Can you work these out from the model? Positions are in its coordinate system, mm. A direction names the side the tool comes from. Give positions to 0.01 mm unless a question says otherwise; leave off trailing zeros. Write each loop counter-clockwise with the first axis right and the second up, starting at its lowest first coordinate (ties: lowest second). Pieces come first, ordered by that corner, then holes. Notation, with made-up numbers: (60.25, 64) - (93.25, 64) arc R17 ccw to (93.25, 80) - close; hole circle Ø7 at (50, 2). An arc over 180 degrees is marked (long way). Use a Markdown table: item, result. Add a question column.
```python
from build123d import *

# Parameters (mm, degrees)
SKETCH1_R           = 18
BOSS_EXTRUDE1_DEPTH = 32.6
SKETCH2_R           = 1.6
CUT_EXTRUDE1_DEPTH  = 42.361334601
CIRPATTERN1_COUNT   = 8
SKETCH3_R           = 11
BOSS_EXTRUDE2_DEPTH = 2
SKETCH4_R           = 4
BOSS_EXTRUDE3_DEPTH = 16
CUT_EXTRUDE2_START  = -15
CUT_EXTRUDE2_DEPTH  = 15


with BuildPart() as part:
    # Sketch1 → Boss-Extrude1 (new body)
    with BuildSketch(Plane.XY):
        Circle(SKETCH1_R)
    extrude(amount=BOSS_EXTRUDE1_DEPTH)

    # Sketch2 → Cut-Extrude1 (cut, through all)
    with BuildSketch(Plane(origin=(0, 0, 0), x_dir=(-1, 0, 0), z_dir=(0, 0, -1))):
        with Locations((0, 14)):
            Circle(SKETCH2_R)
    cut_extrude1 = extrude(amount=-CUT_EXTRUDE1_DEPTH, mode=Mode.SUBTRACT)

    # CirPattern1: Cut-Extrude1 ×8 about axis
    cirpattern1_axis = Axis((0, 0, 0), (0, 0, 1))
    for i in range(1, CIRPATTERN1_COUNT):
        add(cut_extrude1.rotate(cirpattern1_axis, i * 360 / CIRPATTERN1_COUNT), mode=Mode.SUBTRACT)

    # Sketch3 → Boss-Extrude2 (add)
    with BuildSketch(Plane(origin=(0, 0, 0), x_dir=(-1, 0, 0), z_dir=(0, 0, -1))):
        with Locations(Location((0, 0, 0), (0, 0, 180))):
            Circle(SKETCH3_R)
    extrude(amount=BOSS_EXTRUDE2_DEPTH)

    # Sketch4 → Boss-Extrude3 (add)
    with BuildSketch(Plane(origin=(0, 0, -2), x_dir=(-1, 0, 0), z_dir=(0, 0, -1))):
        Circle(SKETCH4_R)
    extrude(amount=BOSS_EXTRUDE3_DEPTH)

    # Sketch5 → Cut-Extrude2 (cut)
    with BuildSketch(Plane(origin=(0, 0, -18), x_dir=(-1, 0, 0), z_dir=(0, 0, -1)).offset(CUT_EXTRUDE2_START)):
        with BuildLine():
            Line((-2.645751311, 3), (2.645751311, 3))
            ThreePointArc((2.645751311, 3), (0, 4), (-2.645751311, 3))
        make_face()
        with BuildLine():
            Line((-2.645751311, -3), (2.645751311, -3))
            ThreePointArc((2.645751311, -3), (0, -4), (-2.645751311, -3))
        make_face()
    extrude(amount=CUT_EXTRUDE2_DEPTH, mode=Mode.SUBTRACT)


solid = part.part
```
Q1. If we mould it in two halves opening along X, with no side actions, what happens to faces 6 (the cylindrical face through (-8.374, -9.418, 16.072)), 7 (the flat face through (0, 0, 32.6)), 8 (the cylindrical face through (-9.418, 8.374, 16.072)), 9 (the cylindrical face through (-2.343, 17.847, 16.072))? For each: released by +X, released by -X, zero draft, split by the parting line, or undercut.
Q2. I'm going to push flat-ended pins straight in: P1, Ø4, axis at x = 9.9, y = 9.9, coming from the -Z side; P2, Ø1.5, axis at y = 13, z = 0, coming from the +X side; P3, Ø0.8, axis at x = 0, y = -3.5, coming from the -Z side. Where does each tip first touch, or does it pass through?
Q3. Suppose I cut it at B-B (x = 0). Please give me the cut outline in (y, z), and give its area (3 significant figures).
Q4. If I drill on probe 1 along Y at (x, z) = (0, 10); probe 2 along Y at (x, z) = (0.5, 22); probe 3 along Z at (x, y) = (-5.5, 3), over which ranges is the centre line in solid material (lowest first)? Write a range as [from, to].
Q5. Suppose I cut it at A-A (y = 0). Please give me the cut outline in (x, z), and give its area (3 significant figures).
Q6. On a 3-axis mill with a long thin cutter (end or side, diameter ignored), from which of +Z, -Z, +X, -X, +Y, -Y can I reach the whole of each face in a straight line? I mean faces 1 (the cylindrical face through (-0.208, -15.586, 16.072)), 2 (the flat face through (0, -3, -10)), 3 (the flat face through (0, 0, -18)), 4 (the flat face through (0, 3, -10)), 5 (the flat face through (0, 5, -2)). Say none if no direction works.
Q7. Suppose I cut it at C-C (z = 14). Give the number of separate pieces and of enclosed holes in the cut face, and give its area (3 significant figures).
Q8. Suppose I cut it at D-D (x = -14). Please give me the cut outline in (y, z), and give its area (3 significant figures).
Derived:
| question | item | result |
|---|---|---|
| 1 | face 6 | undercut |
| 1 | face 7 | zero draft |
| 1 | face 8 | undercut |
| 1 | face 9 | split by the parting line |
| 2 | P1 | z = 0 |
| 2 | P2 | x = 13.19 |
| 2 | P3 | z = -3 |
| 3 | outline | (-18, 0) - (-15.6, 0) - (-15.6, 32.6) - (-18, 32.6) - close; (-12.4, 0) - (-11, 0) - (-11, -2) - (-4, -2) - (-4, -3) - (-3, -3) - (-3, -18) - (3, -18) - (3, -3) - (4, -3) - (4, -2) - (11, -2) - (11, 0) - (12.4, 0) - (12.4, 32.6) - (-12.4, 32.6) - close; (15.6, 0) - (18, 0) - (18, 32.6) - (15.6, 32.6) - close |
| 3 | area | 1,110 mm² |
| 4 | probe 1 | [-18, -15.6], [-12.4, 12.4], [15.6, 18] |
| 4 | probe 2 | [-17.99, -15.52], [-12.48, 12.48], [15.52, 17.99] |
| 4 | probe 3 | [-2, 32.6] |
| 5 | outline | (-18, 0) - (-15.6, 0) - (-15.6, 32.6) - (-18, 32.6) - close; (-12.4, 0) - (-11, 0) - (-11, -2) - (-4, -2) - (-4, -18) - (4, -18) - (4, -2) - (11, -2) - (11, 0) - (12.4, 0) - (12.4, 32.6) - (-12.4, 32.6) - close; (15.6, 0) - (18, 0) - (18, 32.6) - (15.6, 32.6) - close |
| 5 | area | 1,140 mm² |
| 6 | face 1 | +Z, -Z |
| 6 | face 2 | -Z, +X, -X, -Y |
| 6 | face 3 | -Z, +X, -X, +Y, -Y |
| 6 | face 4 | -Z, +X, -X, +Y |
| 6 | face 5 | -Z |
| 7 | separate pieces | 1 |
| 7 | enclosed holes | 8 |
| 7 | area | 954 mm² |
| 8 | outline | (-11.31, 0) - (-1.6, 0) - (-1.6, 32.6) - (-11.31, 32.6) - close; (1.6, 0) - (11.31, 0) - (11.31, 32.6) - (1.6, 32.6) - close |
| 8 | area | 633 mm² |
